Work out the finished part from the listing and answer in its coordinate system (mm). A direction names the side the tool comes from. Give positions to 0.01 mm unless a question says otherwise; leave off trailing zeros. Loops run counter-clockwise (first coordinate to the right, second up) from the corner with the lowest first, then second, coordinate; pieces in that order, holes last. Notation, with made-up numbers: M 33.5,25 L 53.5,25 A33 ccw 53.5,57 Z; hole C 56.5,-34.75 d2. An arc over 180 degrees is marked long. Answer in a Markdown table with one row per item. Add a question column.
from build123d import *

# Parameters (mm, degrees)
SKETCH1_W               = 38.5
SKETCH1_H               = 20.85
BOSS_EXTRUDE1_DEPTH     = 9
SKETCH2_W               = 5
SKETCH2_H               = 19.65
BOSS_EXTRUDE2_DEPTH     = 9
SKETCH3_R               = 7.5
BOSS_EXTRUDE3_DEPTH     = 4.5
SKETCH4_W               = 23.2
SKETCH4_H               = 13
CUT_EXTRUDE1_DEPTH      = 18.85
SKETCH5_R               = 5
CUT_EXTRUDE3_DEPTH      = 4
SKETCH6_W               = 1.4
SKETCH6_H               = 13
CUT_EXTRUDE5_DEPTH      = 5.8
CUT_EXTRUDE6_DEPTH      = 35.351710292
CUT_EXTRUDE6_DEPTH_BACK = 35.351710292
SKETCH7_W               = 10.4
SKETCH7_H               = 4
SKETCH8_R               = 0.8
CUT_EXTRUDE7_DEPTH      = 8
SKETCH9_R               = 0.8
CUT_EXTRUDE8_DEPTH      = 8
SKETCH10_R              = 0.8
CUT_EXTRUDE9_DEPTH      = 10
SKETCH11_R              = 0.8
CUT_EXTRUDE10_DEPTH     = 10
BOSS_EXTRUDE4_DEPTH     = 9
SKETCH13_W              = 6
SKETCH13_H              = 13
CUT_EXTRUDE11_DEPTH     = 9.85
SKETCH14_R              = 0.8
CUT_EXTRUDE13_DEPTH     = 6


with BuildPart() as part:
    # Sketch1 → Boss-Extrude1 (new, symmetric)
    with BuildSketch(Plane.XY):
        with Locations((-2.75, -5.275)):
            Rectangle(SKETCH1_W, SKETCH1_H)
    extrude(amount=BOSS_EXTRUDE1_DEPTH, both=True)

    # Sketch2 → Boss-Extrude2 (add, symmetric)
    with BuildSketch(Plane.XY):
        with Locations((-19.5, 14.975)):
            Rectangle(SKETCH2_W, SKETCH2_H)
    extrude(amount=BOSS_EXTRUDE2_DEPTH, both=True)

    # Sketch3 → Boss-Extrude3 (add)
    with BuildSketch(Plane(origin=(0, -20.2, 0), x_dir=(1, 0, 0), z_dir=(0, 1, 0))):
        with Locations(Location((5.5, 0, 0), (0, 0, 270))):
            Circle(SKETCH3_R)
    extrude(amount=BOSS_EXTRUDE3_DEPTH)

    # Sketch4 → Cut-Extrude1 (cut)
    with BuildSketch(Plane(origin=(0, 5.15, 0), x_dir=(1, 0, 0), z_dir=(0, 1, 0))):
        Rectangle(SKETCH4_W, SKETCH4_H)
    extrude(amount=-CUT_EXTRUDE1_DEPTH, mode=Mode.SUBTRACT)

    # Sketch5 → Cut-Extrude3 (cut)
    with BuildSketch(Plane(origin=(0, -20.2, 0), x_dir=(1, 0, 0), z_dir=(0, 1, 0))):
        with Locations(Location((5.5, 0, 0), (0, 0, 270))):
            Circle(SKETCH5_R)
    extrude(amount=CUT_EXTRUDE3_DEPTH, mode=Mode.SUBTRACT)

    # Sketch6 → Cut-Extrude5 (cut)
    with BuildSketch(Plane(origin=(0, -13.7, 0), x_dir=(1, 0, 0), z_dir=(0, 1, 0))):
        with Locations((12.3, 0)):
            Rectangle(SKETCH6_W, SKETCH6_H)
    extrude(amount=CUT_EXTRUDE5_DEPTH, mode=Mode.SUBTRACT)

    # Sketch7 → Cut-Extrude6 (cut, two sides: drawn at the far end of the back side and taken through both)
    with BuildSketch(Plane.XY.offset(-CUT_EXTRUDE6_DEPTH_BACK)):
        with Locations((-16.8, -11.7)):
            Rectangle(SKETCH7_W, SKETCH7_H)
    extrude(amount=CUT_EXTRUDE6_DEPTH + CUT_EXTRUDE6_DEPTH_BACK, mode=Mode.SUBTRACT)

    # Sketch8 → Cut-Extrude7 (cut)
    with BuildSketch(Plane(origin=(0, 5.15, 0), x_dir=(1, 0, 0), z_dir=(0, 1, 0))):
        with Locations(Location((-13.75, 0, 0), (0, 0, 270))):
            Circle(SKETCH8_R)
    extrude(amount=-CUT_EXTRUDE7_DEPTH, mode=Mode.SUBTRACT)

    # Sketch9 → Cut-Extrude8 (cut)
    with BuildSketch(Plane(origin=(0, 5.15, 0), x_dir=(1, 0, 0), z_dir=(0, 1, 0))):
        with Locations(Location((13.75, 0, 0), (0, 0, 270))):
            Circle(SKETCH9_R)
    extrude(amount=-CUT_EXTRUDE8_DEPTH, mode=Mode.SUBTRACT)

    # Sketch10 → Cut-Extrude9 (cut)
    with BuildSketch(Plane(origin=(0, 24.8, 0), x_dir=(1, 0, 0), z_dir=(0, 1, 0))):
        with Locations(Location((-19.5, -4.5, 0), (0, 0, 270))):
            Circle(SKETCH10_R)
    extrude(amount=-CUT_EXTRUDE9_DEPTH, mode=Mode.SUBTRACT)

    # Sketch11 → Cut-Extrude10 (cut)
    with BuildSketch(Plane(origin=(0, 24.8, 0), x_dir=(1, 0, 0), z_dir=(0, 1, 0))):
        with Locations(Location((-19.5, 4.5, 0), (0, 0, 270))):
            Circle(SKETCH11_R)
    extrude(amount=-CUT_EXTRUDE10_DEPTH, mode=Mode.SUBTRACT)

    # Sketch12 → Boss-Extrude4 (add, symmetric)
    with BuildSketch(Plane.XY):
        Polygon((-17, 5.15), (-11, 5.15), (-17, 14.975), align=None)
    extrude(amount=BOSS_EXTRUDE4_DEPTH, both=True)

    # Sketch13 → Cut-Extrude11 (cut)
    with BuildSketch(Plane(origin=(0, 15, 0), x_dir=(1, 0, 0), z_dir=(0, 1, 0))):
        with Locations((-14, 0)):
            Rectangle(SKETCH13_W, SKETCH13_H)
    extrude(amount=-CUT_EXTRUDE11_DEPTH, mode=Mode.SUBTRACT)

    # Sketch14 → Cut-Extrude13 (cut)
    with BuildSketch(Plane(origin=(-22, 0, 0), x_dir=(0, 0, -1), z_dir=(1, 0, 0))):
        with Locations((-4.5, -4.5)):
            Circle(SKETCH14_R)
        with Locations((4.5, -4.5)):
            Circle(SKETCH14_R)
        with Locations(Location((-4.5, 4.5, 0), (0, 0, 125.659087696))):
            Circle(SKETCH14_R)
        with Locations(Location((4.5, 4.5, 0), (0, 0, 125.659087696))):
            Circle(SKETCH14_R)
    extrude(amount=CUT_EXTRUDE13_DEPTH, mode=Mode.SUBTRACT)


solid = part.part
(1) Consider line 1 along Y through (x, z) = (-15, 3.5); line 2 along X through (y, z) = (-0.75, 0); line 3 along X through (y, z) = (19.75, -4.5). Determine where each line is inside the solid, lowest interval first. Write a range as from..to.
(2) Section D-D, the plane x = -13.75 is taken. Determine the outline of the cut face in (y, z), and give its area (3 significant figures).
(3) Each of these flat-tipped pins is pushed along its axis until it touches: P1, Ø5, axis at x = 1.5, z = 6.5, coming from the +Y side; P2, Ø1.3, axis at x = -13.75, z = 0, coming from the -Y side; P3, Ø0.8, axis at x = -19.5, z = -4, coming from the +Y side; P4, Ø1, axis at x = 5.5, z = 4, coming from the -Y side. Where does it stop, or does it pass through?
(4) Section A-A, the plane y = 4.5 is taken. Determine the outline of the cut face in (x, z), and give its area (3 significant figures).
(5) Which of the six approach directions +Z, -Z, +X, -X, +Y, -Y give full straight-line access (tool end or side, diameter ignored) to faces 1 (the face through (-16, -4.5, -4.5)), 2 (the face through (6, -16.2, 0)), 3 (the face through (-11.6, -12, 8)), 4 (the face through (-12.957, 1.206, -0.104)), 5 (the face through (12, 5.15, 0))?
(6) Section C-C, the plane x = -19.5 is taken. Determine the outline of the cut face in (y, z), and give its area (3 significant figures).
(7) The mould has two halves that part along Y. Classify faces 6 (the face through (-14, -2.85, 0)), 7 (the face through (-17, 15, 0)), 8 (the face through (-19.04, -4.99, -3.87)): pulls with the +Y half, pulls with the -Y half, needs draft (parallel to the pull), parting line crosses it, or undercut.
Numbers:
| question | item | result |
|---|---|---|
| 1 | line 1 | y = -15.7..-13.7, -9.7..5.15 |
| 1 | line 2 | x = -22..-14.55, -12.95..-11.6, 11.6..12.95, 14.55..16.5 |
| 1 | line 3 | x = -22..-20.3, -18.7..-17 |
| 2 | outline | M -15.7,-9 L -13.7,-9 L -13.7,9 L -15.7,9 Z; M -9.7,-9 L 9.65,-9 L 9.65,-6.5 L 5.15,-6.5 L 5.15,-0.8 L -2.85,-0.8 L -2.85,0.8 L 5.15,0.8 L 5.15,6.5 L 9.65,6.5 L 9.65,9 L -9.7,9 Z |
| 2 | area | 313 mm² |
| 3 | P1 | stops at y = 5.15 |
| 3 | P2 | stops at y = -15.7 |
| 3 | P3 | stops at y = 24.8 |
| 3 | P4 | stops at y = -16.2 |
| 4 | outline | M -22,-9 L 16.5,-9 L 16.5,9 L -22,9 L -22,5.3 L -16,5.3 L -16,3.7 L -22,3.7 L -22,-3.7 L -16,-3.7 L -16,-5.3 L -22,-5.3 Z; hole C -13.75,0 d1.6; hole M -11.6,-6.5 L 11.6,-6.5 L 11.6,6.5 L -11.6,6.5 Z; hole C 13.75,0 d1.6 |
| 4 | area | 368 mm² |
| 5 | face 1 | -X |
| 5 | face 2 | -Y |
| 5 | face 3 | +Z, -Z, -X |
| 5 | face 4 | +Y |
| 5 | face 5 | +Z, -Z, +X, +Y |
| 6 | outline | M -15.7,-9 L -13.7,-9 L -13.7,9 L -15.7,9 Z; M -9.7,-9 L 24.8,-9 L 24.8,-5.3 L 14.8,-5.3 L 14.8,-3.7 L 24.8,-3.7 L 24.8,3.7 L 14.8,3.7 L 14.8,5.3 L 24.8,5.3 L 24.8,9 L -9.7,9 Z; hole C -4.5,-4.5 d1.6; hole C -4.5,4.5 d1.6; hole C 4.5,-4.5 d1.6; hole C 4.5,4.5 d1.6 |
| 6 | area | 617 mm² |
| 7 | face 6 | pulls with the +Y half |
| 7 | face 7 | needs draft |
| 7 | face 8 | undercut |
